Model file for the job. Use its own axes, mm. A direction names the side the tool comes from. Round coordinates to 2 decimals unless told otherwise and drop trailing zeros. Order: outer loops, then holes, each group sorted by start corner. A loop starts at its lowest first (then second) coordinate and runs counter-clockwise, first axis right, second up. Notation, with made-up numbers: M -10.75,57.5 L 38.25,57.5 A10 ccw 38.25,61.5 Z; hole C 12.25,77 d4. An arc over 180 degrees is marked long. Return JSON: item names as keys, results as strings. Group by question number.
Item 1: Slice it at A-A on y = -47. Write the cut outline in (x, z).
Item 2: Probe line 1 along Y through (x, z) = (-82, 2.6); line 2 along X through (y, z) = (104.5, 2.45); line 3 along X through (y, z) = (88.5, 0.65). List the from-to ranges inside material, lowest first.
Item 3: Which spindle directions (+Z, -Z, +X, -X, +Y, -Y) get a long thin tool onto all of the face, cutting with end or side? Do faces 1 (the face through (-1, 109.5, 2)), 2 (the face through (-29.7, -59.2, 2.5)). Say none if no direction does.
Item 4: Slice it at C-C on z = 2.25. Give the number of separate pieces and of enclosed holes in the cut face, then the cut area to 3 significant figures.
Item 5: Slice it at D-D on y = 76.5. Write the cut outline in (x, z), then the cut area to 3 significant figures.
Item 6: Pin check, flat tip, straight feed: pin 1 Ø4 at (x, y) = (58, 9) entering from +Z. Stop position of the tip, or through.
Item 7: Slice it at B-B on x = -26. Write the cut outline in (y, z), then the cut area to 3 significant figures.
Item 8: Pull direction Y, two halves, no side cores. Call faces 3 (the face through (-35.2, -16.7, 2.5)), 4 (the face through (-1, -109.5, 2)), 5 (the face through (-109.5, -1, 2)), 6 (the face through (-32.814, 0, 3)): pulls with the +Y half, pulls with the -Y half, needs draft (parallel to the pull), parting line crosses it, or undercut.
from build123d import *

# Parameters (mm, degrees)
F0_W     = 219
F0_H     = 219
F0_R     = 1.6
F1_DEPTH = 5
F2_R     = 2.1
F3_DEPTH = 25
F4_R     = 5
F6_DEPTH = 25


with BuildPart() as f1:
    # F0 (on Top) → F1 (new body)
    with BuildSketch(Plane.XY):
        Rectangle(F0_W, F0_H)
        with Locations((-104.5, -104.5)):
            Circle(F0_R, mode=Mode.SUBTRACT)
        with Locations((104.5, -104.5)):
            Circle(F0_R, mode=Mode.SUBTRACT)
        with Locations((-104.5, 0)):
            Circle(F0_R, mode=Mode.SUBTRACT)
        with Locations((-104.5, 104.5)):
            Circle(F0_R, mode=Mode.SUBTRACT)
        with Locations((104.5, 0)):
            Circle(F0_R, mode=Mode.SUBTRACT)
        with Locations((104.5, 104.5)):
            Circle(F0_R, mode=Mode.SUBTRACT)
    extrude(amount=F1_DEPTH)

    # F2 (on face) → F3 (cut)
    with BuildSketch(Plane.XY.offset(5)):
        with Locations((-82, -54.5)):
            Circle(F2_R)
        with Locations((-58, -54.5)):
            Circle(F2_R)
        with Locations((-58, -36.5)):
            Circle(F2_R)
        with Locations((-82, -36.5)):
            Circle(F2_R)
        with Locations((-82, 36.5)):
            Circle(F2_R)
        with Locations((-82, 54.5)):
            Circle(F2_R)
        with Locations((-58, 54.5)):
            Circle(F2_R)
        with Locations((-58, 36.5)):
            Circle(F2_R)
        with Locations((14.5, -10)):
            Circle(F2_R)
        with Locations((58, -9)):
            Circle(F2_R)
        with Locations((82, -9)):
            Circle(F2_R)
        with Locations((82, 9)):
            Circle(F2_R)
        with Locations((58, 9)):
            Circle(F2_R)
        with Locations((14.5, 10)):
            Circle(F2_R)
    extrude(amount=-F3_DEPTH, mode=Mode.SUBTRACT)

    # F4
    f4_edges = [f1.edges().sort_by_distance(p)[0] for p in [
        (109.5, 109.5, 2.5),
        (109.5, -109.5, 2.5),
        (-109.5, -109.5, 2.5),
        (-109.5, 109.5, 2.5),
    ]]
    fillet(f4_edges, radius=F4_R)

    # F5 (on face) → F6 (cut)
    with BuildSketch(Plane.XY.offset(5)):
        with BuildLine():
            Line((-5.656854, -35.156854), (-54.343146, -83.843146))
            ThreePointArc((-54.343146, -83.843146), (-56.077328, -92.561467), (-48.686292, -97.5))
            Line((-48.686292, -97.5), (48.686292, -97.5))
            ThreePointArc((48.686292, -97.5), (56.077328, -92.561467), (54.343146, -83.843146))
            Line((54.343146, -83.843146), (5.656854, -35.156854))
            ThreePointArc((5.656854, -35.156854), (0, -32.813708), (-5.656854, -35.156854))
        make_face()
        with BuildLine():
            Line((5.656854, 35.156854), (54.343146, 83.843146))
            ThreePointArc((54.343146, 83.843146), (56.077328, 92.561467), (48.686292, 97.5))
            Line((48.686292, 97.5), (-48.686292, 97.5))
            ThreePointArc((-48.686292, 97.5), (-56.077328, 92.561467), (-54.343146, 83.843146))
            Line((-54.343146, 83.843146), (-5.656854, 35.156854))
            ThreePointArc((-5.656854, 35.156854), (0, 32.813708), (5.656854, 35.156854))
        make_face()
        with BuildLine():
            Line((-89.5, -19), (-40.814, -19))
            ThreePointArc((-40.814, -19), (-35.157146, -16.656854), (-32.814, -11))
            Line((-32.814, -11), (-32.814, 11))
            ThreePointArc((-32.814, 11), (-35.157146, 16.656854), (-40.814, 19))
            Line((-40.814, 19), (-89.5, 19))
            ThreePointArc((-89.5, 19), (-95.156854, 16.656854), (-97.5, 11))
            Line((-97.5, 11), (-97.5, -11))
            ThreePointArc((-97.5, -11), (-95.156854, -16.656854), (-89.5, -19))
        make_face()
    extrude(amount=-F6_DEPTH, mode=Mode.SUBTRACT)


solid = f1.part
Output values:
{
 "1": {"outline": "M -109.5,0 L -17.5,0 L -17.5,5 L -109.5,5 Z; M 17.5,0 L 109.5,0 L 109.5,5 L 17.5,5 Z"},
 "2": {"line 1": "-109.5 to -56.6, -52.4 to -38.6, -34.4 to -19, 19 to 34.4, 38.6 to 52.4, 56.6 to 109.5", "line 2": "-109.5 to -106.1, -102.9 to 102.9, 106.1 to 109.5", "line 3": "-109.5 to -56.62, 56.62 to 109.5"},
 "3": {"face 1": "+Z, -Z, +X, -X, +Y", "face 2": "+Z, -Z"},
 "4": {"separate pieces": "1", "enclosed holes": "23", "area": "36,400 mm²"},
 "5": {"outline": "M -109.5,0 L -47,0 L -47,5 L -109.5,5 Z; M 47,0 L 109.5,0 L 109.5,5 L 47,5 Z", "area": "625 mm²"},
 "6": {"pin 1": "through"},
 "7": {"outline": "M -109.5,0 L -97.5,0 L -97.5,5 L -109.5,5 Z; M -55.5,0 L 55.5,0 L 55.5,5 L -55.5,5 Z; M 97.5,0 L 109.5,0 L 109.5,5 L 97.5,5 Z", "area": "675 mm²"},
 "8": {"face 3": "undercut", "face 4": "pulls with the -Y half", "face 5": "needs draft", "face 6": "undercut"}
}
